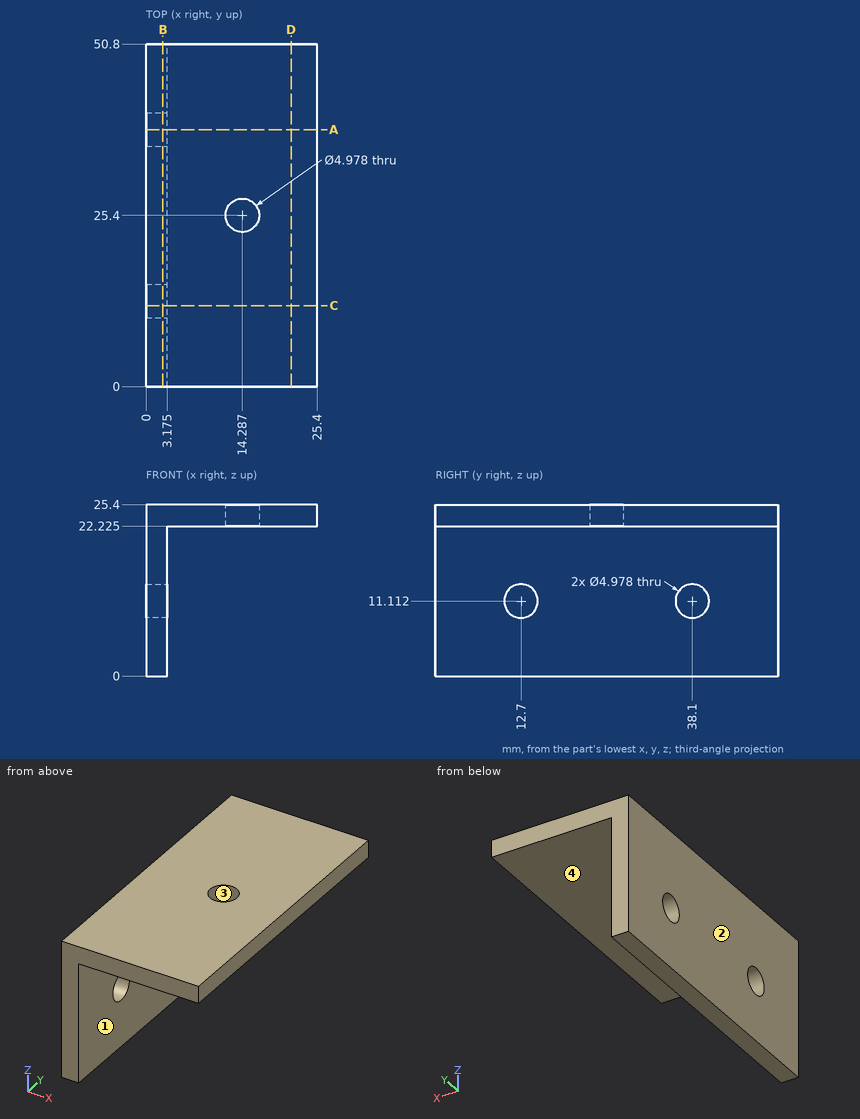
Job drawing, mm, ordinate dimensions from the low corner. One solid piece. Give positions to 0.01 mm unless a question says otherwise; leave off trailing zeros. Loops run counter-clockwise (first coordinate to the right, second up) from the corner with the lowest first, then second, coordinate; pieces in that order, holes last. Notation, with made-up numbers: M -13.75,-7.75 L 5.25,-7.75 A25 cw 5.25,6.25 Z; hole C 46.25,-14 d3. An arc over 180 degrees is marked long. Return JSON: item names as keys, results as strings.
1) Saw through at D-D, the plane x = 21.5. List the corners of the cut face in (y, z) (1 decimal), then the cut area to 3 significant figures.
Calculated:
{"outline": "M 0,22.2 L 50.8,22.2 L 50.8,25.4 L 0,25.4 Z", "area": "161 mm2"}
2) Pull direction X, two halves, no side cores. Call the marked faces 1, 2, 3 and 4: released by +X, released by -X, zero draft, split by the parting line, or undercut.
Calculated:
{"face 1": "released by +X", "face 2": "released by -X", "face 3": "undercut", "face 4": "zero draft"}
3) Flat gauge pins, fed straight in: pin 1 Ø8 at (y, z) = (12.7, 11.11) entering from -X; pin 2 Ø6.5 at (y, z) = (38.1, 11.11) entering from +X (1 decimal); pin 3 Ø4.5 at (x, y) = (14.29, 25.4) entering from -Z. Where does each tip first touch, or does it go through?
Calculated:
{"pin 1": "stops at x = 0", "pin 2": "stops at x = 3.2", "pin 3": "passes through"}
4) Saw through at C-C, the plane y = 12. List the corners of the cut face in (x, z) (1 decimal).
Calculated:
{"outline": "M 0,0 L 3.2,0 L 3.2,8.7 L 0,8.7 Z; M 0,13.5 L 3.2,13.5 L 3.2,22.2 L 25.4,22.2 L 25.4,25.4 L 0,25.4 Z"}
5) Drill centre lines: line 1 (Z direction, x = 12, y = 37) (1 decimal); line 2 (X direction, y = 17.5, z = 3) (1 decimal); line 3 (X direction, y = 24.5, z = 24.25) (1 decimal). Where is each one in solid material? Low to high.
Calculated:
{"line 1": "z = 22.2 to 25.4", "line 2": "x = 0 to 3.2", "line 3": "x = 0 to 12, 16.6 to 25.4"}
6) Saw through at B-B, the plane x = 2.5. List the corners of the cut face in (y, z).
Calculated:
{"outline": "M 0,0 L 50.8,0 L 50.8,25.4 L 0,25.4 Z; hole C 12.7,11.11 d4.98; hole C 38.1,11.11 d4.98"}
7) Saw through at A-A, the plane y = 38.1. List the corners of the cut face in (x, z) (1 decimal).
Calculated:
{"outline": "M 0,0 L 3.2,0 L 3.2,8.6 L 0,8.6 Z; M 0,13.6 L 3.2,13.6 L 3.2,22.2 L 25.4,22.2 L 25.4,25.4 L 0,25.4 Z"}
